Work out the finished part from the listing and answer in its coordinate system (mm). A direction names the side the tool comes from. Give positions to 0.01 mm unless a question says otherwise; leave off trailing zeros. Loops run counter-clockwise (first coordinate to the right, second up) from the corner with the lowest first, then second, coordinate; pieces in that order, holes last. Notation, with made-up numbers: (63, 74) -> (71, 74) arc R24 ccw to (71, 108) -> close; hole circle Ø11 at (14, 86). An arc over 180 degrees is marked (long way). Answer as CSV lines item,"result". Start each with the question number.
1. Find section A-A, the plane x = 0. Give the vertices of the cut face in (y, z).
2. Find the intervals of material crossed by line 1 along Y through (x, z) = (0, 0.8); line 2 along Y through (x, z) = (-2, 3.45); line 3 along X through (y, z) = (-2, 1.1), in increasing order.
3. Find section C-C, the plane y = -1. Give the vertices of the cut face in (x, z).
4. Find section B-B, the plane z = 2.3. Give the vertices of the cut face in (x, y).
5. Find section D-D, the plane x = -8. Give the vertices of the cut face in (y, z), and give its area (3 significant figures).
6. Flat-ended cylindrical pins translate along their axes: pin 1 Ø2 at (x, y) = (16.5, -12.5) entering from -Z; pin 2 Ø1 at (y, z) = (-2.5, 1) entering from -X; pin 3 Ø3 at (x, y) = (0, 0) entering from +Z; pin 4 Ø1 at (y, z) = (-2, 3) entering from +X. Find the tip coordinate at first contact, or state that the pin passes through.
7. Determine the mould class of faces 3 (the face through (0, 3.377, 3)), 4 (the face through (18.66, -10.98, 0.49)), 5 (the face through (-18.66, 10.98, 0.49)), 6 (the face through (4.5, 0.3, 4)) for opening direction Y: +Y half, -Y half, draft (parallel to the pull), parting line (faces both ways), or undercut.
8. A tool of negligible diameter and unlimited length cuts with its end or side. For faces 1 (the face through (2.911, -1.712, 2.521)), 2 (the face through (5, 0, 0)), from which of +Z, -Z, +X, -X, +Y, -Y can it reach the whole face along a straight path? Write none if from no direction.
from build123d import *

# Parameters (mm, degrees)
PAD_DEPTH       = 4
POCKET_DEPTH    = 3
SKETCH002_R     = 2
POCKET001_DEPTH = 5
CHAMFER_SIZE    = 3


with BuildPart() as part:
    # Sketch → Pad (new body)
    with BuildSketch(Plane.XY):
        Polygon((12.5, 21.650635), (-12.5, 21.650635), (-25, 0), (-12.5, -21.650635), (12.5, -21.650635), (25, 0), align=None)
    extrude(amount=PAD_DEPTH)

    # Sketch001 (on Face8 of Pad) → Pocket (cut)
    with BuildSketch(Plane.XY.offset(4)):
        Polygon((1.95, 3.377499), (-1.95, 3.377499), (-3.9, 0), (-1.95, -3.377499), (1.95, -3.377499), (3.9, 0), align=None)
    extrude(amount=-POCKET_DEPTH, mode=Mode.SUBTRACT)

    # Sketch002 (on Face15 of Pocket) → Pocket001 (cut)
    with BuildSketch(Plane.XY.offset(1)):
        Circle(SKETCH002_R)
    extrude(amount=-POCKET001_DEPTH, mode=Mode.SUBTRACT)

    # Chamfer
    chamfer_edges = [part.edges().sort_by_distance(p)[0] for p in [
        (-18.75, 10.825318, 4),
        (-18.75, -10.825318, 4),
        (0, -21.650635, 4),
        (18.75, -10.825318, 4),
        (18.75, 10.825318, 4),
        (0, 21.650635, 4),
    ]]
    chamfer(chamfer_edges, length=CHAMFER_SIZE)


solid = part.part
Resolved:
1,outline,"(-21.65, 0) -> (-2, 0) -> (-2, 1) -> (-3.38, 1) -> (-3.38, 4) -> (-18.65, 4) -> (-21.65, 1) -> close; (2, 0) -> (21.65, 0) -> (21.65, 1) -> (18.65, 4) -> (3.38, 4) -> (3.38, 1) -> (2, 1) -> close"
2,line 1,"y = -21.65 to -2, 2 to 21.65"
2,line 2,"y = -19.2 to -3.29, 3.29 to 19.2"
2,line 3,"x = -23.73 to -2.75, 2.75 to 23.73"
3,outline,"(-24.42, 0) -> (-1.73, 0) -> (-1.73, 1) -> (-3.32, 1) -> (-3.32, 4) -> (-20.96, 4) -> (-24.42, 1) -> close; (1.73, 0) -> (24.42, 0) -> (24.42, 1) -> (20.96, 4) -> (3.32, 4) -> (3.32, 1) -> (1.73, 1) -> close"
4,outline,"(-23.5, 0) -> (-11.75, -20.35) -> (11.75, -20.35) -> (23.5, 0) -> (11.75, 20.35) -> (-11.75, 20.35) -> close; hole (-3.9, 0) -> (-1.95, -3.38) -> (1.95, -3.38) -> (3.9, 0) -> (1.95, 3.38) -> (-1.95, 3.38) -> close"
5,outline,"(-21.65, 0) -> (21.65, 0) -> (21.65, 1) -> (18.65, 4) -> (-18.65, 4) -> (-21.65, 1) -> close"
5,area,"164 mm^2"
6,pin 1,"stops at z = 0"
6,pin 2,"stops at x = -23.85"
6,pin 3,"passes through"
6,pin 4,"stops at x = 22.18"
7,face 3,"undercut"
7,face 4,"-Y half"
7,face 5,"+Y half"
7,face 6,"draft"
8,face 1,"+Z"
8,face 2,"-Z, +X, -X, +Y, -Y"
